from build123d import *

# Parameters (mm, degrees)
SKETCH1_W           = 7
SKETCH1_H           = 7
BOSS_EXTRUDE1_DEPTH = 40
SKETCH2_R           = 1.5
CUT_EXTRUDE1_DEPTH  = 41
SKETCH3_W           = 5.5
SKETCH3_H           = 2
CUT_EXTRUDE2_DEPTH  = 41


with BuildPart() as part:
    # Sketch1 → Boss-Extrude1 (new body)
    with BuildSketch(Plane(origin=(0, 0, 0), x_dir=(1, 0, 0), z_dir=(0, 1, 0))):
        Rectangle(SKETCH1_W, SKETCH1_H)
    extrude(amount=BOSS_EXTRUDE1_DEPTH)

    # Sketch2 → Cut-Extrude1 (cut)
    with BuildSketch(Plane(origin=(0, 40, 0), x_dir=(1, 0, 0), z_dir=(0, 1, 0))):
        Circle(SKETCH2_R)
    extrude(amount=-CUT_EXTRUDE1_DEPTH, mode=Mode.SUBTRACT)

    # Sketch3 → Cut-Extrude2 (cut)
    with BuildSketch(Plane.XY.offset(3.5)):
        with Locations((0, 3)):
            Rectangle(SKETCH3_W, SKETCH3_H)
        with Locations((0, 37)):
            Rectangle(SKETCH3_W, SKETCH3_H)
    extrude(amount=-CUT_EXTRUDE2_DEPTH, mode=Mode.SUBTRACT)


solid = part.part
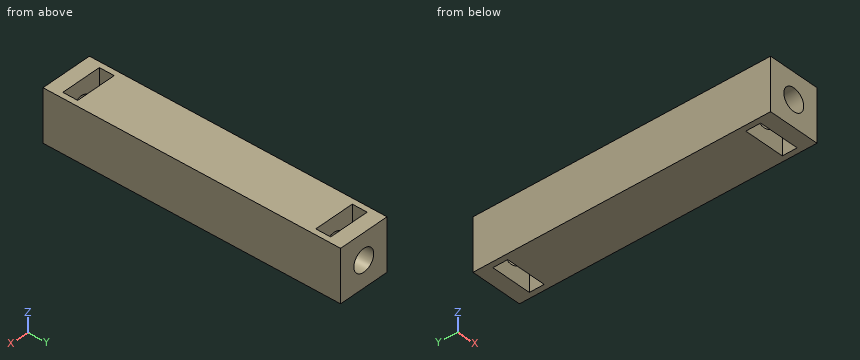
Geometry check sheet. Reference: the model listing, model coordinates, mm. Give positions to 0.01 mm unless a question says otherwise; leave off trailing zeros. Write each loop counter-clockwise with the first axis right and the second up, starting at its lowest first coordinate (ties: lowest second). Pieces come first, ordered by that corner, then holes. Notation, with made-up numbers: M 18,28.5 L 41,28.5 A30 cw 41,60.5 Z; hole C 45.5,-24.5 d10. An arc over 180 degrees is marked long. Answer as CSV lines item,"result". Start each with the question number.
Q1. Material ranges on L1, parallel to Y at x = 1.5, z = 2; L2, parallel to X at y = 1.25, z = 0, recorded low to high.
Q2. Section check C-C, the plane x = -2.25. Record the cut outline in (y, z), then the cut area to 3 significant figures.
Q3. Section check A-A, the plane z = 0. Record the cut outline in (x, y), then the cut area to 3 significant figures.
Q4. Section check D-D, the plane y = 20. Record the cut outline in (x, z), then the cut area to 3 significant figures.
Q5. Go/stop test with a flat-tipped pin: pin 1 (1.8 mm diameter, centred on x = 0, z = 0, fed in from -Y). Record where the tip stops, or that it passes through.
Q6. Section check B-B, the plane x = 0. Record the cut outline in (y, z).
Geometry says:
1,L1,"0 to 2, 4 to 36, 38 to 40"
1,L2,"-3.5 to -1.5, 1.5 to 3.5"
2,outline,"M 0,-3.5 L 2,-3.5 L 2,3.5 L 0,3.5 Z; M 4,-3.5 L 36,-3.5 L 36,3.5 L 4,3.5 Z; M 38,-3.5 L 40,-3.5 L 40,3.5 L 38,3.5 Z"
2,area,"252 mm^2"
3,outline,"M -3.5,0 L -1.5,0 L -1.5,2 L -2.75,2 L -2.75,4 L -1.5,4 L -1.5,36 L -2.75,36 L -2.75,38 L -1.5,38 L -1.5,40 L -3.5,40 Z; M 1.5,0 L 3.5,0 L 3.5,40 L 1.5,40 L 1.5,38 L 2.75,38 L 2.75,36 L 1.5,36 L 1.5,4 L 2.75,4 L 2.75,2 L 1.5,2 Z"
3,area,"150 mm^2"
4,outline,"M -3.5,-3.5 L 3.5,-3.5 L 3.5,3.5 L -3.5,3.5 Z; hole C 0,0 d3"
4,area,"41.9 mm^2"
5,pin 1,"through"
6,outline,"M 0,-3.5 L 2,-3.5 L 2,-1.5 L 0,-1.5 Z; M 0,1.5 L 2,1.5 L 2,3.5 L 0,3.5 Z; M 4,-3.5 L 36,-3.5 L 36,-1.5 L 4,-1.5 Z; M 4,1.5 L 36,1.5 L 36,3.5 L 4,3.5 Z; M 38,-3.5 L 40,-3.5 L 40,-1.5 L 38,-1.5 Z; M 38,1.5 L 40,1.5 L 40,3.5 L 38,3.5 Z"
